```python
from build123d import *

# Parameters (mm, degrees)
SKETCH1_R           = 98.425
SKETCH1_R_2         = 25.4
BOSS_EXTRUDE1_DEPTH = 7.62
BOSS_EXTRUDE2_DEPTH = 25.4
SKETCH5_R           = 5.2578
CUT_EXTRUDE3_DEPTH  = 19.05
SKETCH6_R           = 3.175
CUT_EXTRUDE4_DEPTH  = 12.7
CIRPATTERN1_COUNT   = 12
CIRPATTERN2_COUNT   = 4
SKETCH8_R           = 1.7526
CUT_EXTRUDE6_DEPTH  = 34.02
CIRPATTERN3_COUNT   = 4


with BuildPart() as part:
    # Sketch1 → Boss-Extrude1 (new body)
    with BuildSketch(Plane(origin=(0, 0, 0), x_dir=(1, 0, 0), z_dir=(0, 1, 0))):
        Circle(SKETCH1_R)
        Circle(SKETCH1_R_2, mode=Mode.SUBTRACT)
    extrude(amount=BOSS_EXTRUDE1_DEPTH)

    # Sketch2 → Boss-Extrude2 (add)
    with BuildSketch(Plane.XZ):
        with BuildLine():
            Line((-14.092921054, 83.751577801), (-14.875155352, 97.29445194))
            ThreePointArc((-14.875155352, 97.29445194), (-0.679076319, 98.422657353), (13.531218764, 97.490444372))
            Line((13.531218764, 97.490444372), (13.333659481, 80.753245397))
            ThreePointArc((13.333659481, 80.753245397), (-1.546485964, 71.578862712), (-14.092921054, 83.751577801))
        make_face()
        with BuildLine():
            Line((83.751577801, 14.092921054), (97.29445194, 14.875155352))
            ThreePointArc((97.29445194, 14.875155352), (98.422657353, 0.679076319), (97.490444372, -13.531218764))
            Line((97.490444372, -13.531218764), (80.753245397, -13.333659481))
            ThreePointArc((80.753245397, -13.333659481), (71.578862712, 1.546485964), (83.751577801, 14.092921054))
        make_face()
        with BuildLine():
            Line((14.092921054, -83.751577801), (14.875155352, -97.29445194))
            ThreePointArc((14.875155352, -97.29445194), (0.679076319, -98.422657353), (-13.531218764, -97.490444372))
            Line((-13.531218764, -97.490444372), (-13.333659481, -80.753245397))
            ThreePointArc((-13.333659481, -80.753245397), (1.546485964, -71.578862712), (14.092921054, -83.751577801))
        make_face()
        with BuildLine():
            Line((-83.751577801, -14.092921054), (-97.29445194, -14.875155352))
            ThreePointArc((-97.29445194, -14.875155352), (-98.422657353, -0.679076319), (-97.490444372, 13.531218764))
            Line((-97.490444372, 13.531218764), (-80.753245397, 13.333659481))
            ThreePointArc((-80.753245397, 13.333659481), (-71.578862712, -1.546485964), (-83.751577801, -14.092921054))
        make_face()
    extrude(amount=BOSS_EXTRUDE2_DEPTH)

    # Sketch5 → Cut-Extrude3 (cut)
    with BuildSketch(Plane.XZ.offset(25.4)):
        with Locations((0, 85.725)):
            Circle(SKETCH5_R)
    cut_extrude3 = extrude(amount=-CUT_EXTRUDE3_DEPTH, mode=Mode.SUBTRACT)

    # Sketch6 → Cut-Extrude4 (cut)
    with BuildSketch(Plane(origin=(0, 7.62, 0), x_dir=(1, 0, 0), z_dir=(0, 1, 0))):
        with Locations((-23.830763578, 88.937620456)):
            Circle(SKETCH6_R)
    cut_extrude4 = extrude(amount=-CUT_EXTRUDE4_DEPTH, mode=Mode.SUBTRACT)

    # CirPattern1: Cut-Extrude4 ×12 about axis
    cirpattern1_axis = Axis((0, 0, 0), (0, 1, 0))
    for i in range(1, CIRPATTERN1_COUNT):
        add(cut_extrude4.rotate(cirpattern1_axis, i * 360 / CIRPATTERN1_COUNT), mode=Mode.SUBTRACT)

    # CirPattern2: Cut-Extrude3 ×4 about axis
    cirpattern2_axis = Axis((0, 0, 0), (0, 1, 0))
    for i in range(1, CIRPATTERN2_COUNT):
        add(cut_extrude3.rotate(cirpattern2_axis, i * 360 / CIRPATTERN2_COUNT), mode=Mode.SUBTRACT)

    # Sketch8 → Cut-Extrude6 (cut, through all)
    with BuildSketch(Plane(origin=(0, 7.62, 0), x_dir=(1, 0, 0), z_dir=(0, 1, 0))):
        with Locations((0, 85.725)):
            Circle(SKETCH8_R)
    cut_extrude6 = extrude(amount=-CUT_EXTRUDE6_DEPTH, mode=Mode.SUBTRACT)

    # CirPattern3: Cut-Extrude6 ×4 about axis
    cirpattern3_axis = Axis((0, 0, 0), (0, 1, 0))
    for i in range(1, CIRPATTERN3_COUNT):
        add(cut_extrude6.rotate(cirpattern3_axis, i * 360 / CIRPATTERN3_COUNT), mode=Mode.SUBTRACT)


solid = part.part
```
Model file for the job. Use its own axes, mm. A direction names the side the tool comes from. Coordinates: 2 decimals unless noted, no trailing zeros. Order: outer loops, then holes, each group sorted by start corner. A loop starts at its lowest first (then second) coordinate and runs counter-clockwise, first axis right, second up. Notation, with made-up numbers: (57.5, -11) - (73.5, -11) arc R14 ccw to (73.5, 1) - close; hole circle Ø1 at (74, -22). An arc over 180 degrees is marked (long way). Return JSON: item names as keys, results as strings. Group by question number.
1) Mould opens along X. For faces 1 (the cylindrical face through (-1.284, -12.522, 71.553)), 2 (the flat face through (-86, -6.35, 2)), 3 (the flat face through (20, 7.62, 20)) say: released by +X, released by -X, zero draft, split by the parting line, or undercut.
2) Saw through at B-B, the plane z = -33.5. Write the cut outline in (x, y).
3) Tool access for faces 4 (the cylindrical face through (-62.174, 3.863, 66.323)), 5 (the flat face through (14.48, -12.52, -90.43)), 6 (the flat face through (-2, -6.35, -86)): list every direction of +Z, -Z, +X, -X, +Y, -Y with a clear straight run to the whole face (end or side of a thin tool).
4) Flat gauge pins, fed straight in: P1, Ø3, axis at x = -86.5, z = 1, coming from the -Y side; P2, Ø2, axis at x = 0, z = -85.725, coming from the +Y side; P3, Ø8.5, axis at x = -23.83, z = 88.94, coming from the -Y side; P4, Ø3, axis at y = -1, z = -39.5, coming from the -X side. Where does each tip first touch, or does it go through?
5) Probe line 1 (Z direction, x = 0, y = -19) (3 decimals); line 2 (Y direction, x = 54, z = -31); line 3 (Z direction, x = 2.5, y = -8.5). List the from-to ranges inside material, lowest first. Write a range as from..to.
6) Saw through at A-A, the plane y = -3. Write the cut outline in (x, z) (3 decimals), plus the area to 3 significant figures.
Values found:
{
 "1": {"face 1": "split by the parting line", "face 2": "undercut", "face 3": "zero draft"},
 "2": {"outline": "(-92.55, 0) - (92.55, 0) - (92.55, 7.62) - (-92.55, 7.62) - close"},
 "3": {"face 4": "+Y, -Y", "face 5": "+Z, +X, -Y", "face 6": "-Y"},
 "4": {"P1": "stops at y = -6.35", "P2": "passes through", "P3": "stops at y = 0", "P4": "stops at x = -90.63"},
 "5": {"line 1": "z = -98.425..-90.983, -80.467..-71.495, 71.495..80.467, 90.983..98.425", "line 2": "y = 0..7.62", "line 3": "z = -98.39..-90.35, -81.1..-71.72, 71.72..81.1, 90.35..98.39"},
 "6": {"outline": "(-97.49, 13.531) arc R98.425 ccw to (-97.294, -14.875) - (-83.752, -14.093) arc R14.23 ccw to (-80.753, 13.334) - close; (-14.875, 97.294) - (-14.093, 83.752) arc R14.23 ccw to (13.334, 80.753) - (13.531, 97.49) arc R98.425 ccw to start; (-13.531, -97.49) arc R98.425 ccw to (14.875, -97.294) - (14.093, -83.752) arc R14.23 ccw to (-13.334, -80.753) - close; (80.753, -13.334) - (97.49, -13.531) arc R98.425 ccw to (97.294, 14.875) - (83.752, 14.093) arc R14.23 ccw to start; hole circle Ø3.505 at (-85.725, 0); hole circle Ø3.505 at (0, -85.725); hole circle Ø3.505 at (0, 85.725); hole circle Ø3.505 at (85.725, 0)", "area": "2,610 mm²"}
}
